Design review of the part built by this model. Coordinates are the model's own, in mm. A direction names the side the tool comes from. Give positions to 0.01 mm unless a question says otherwise; leave off trailing zeros. Loops run counter-clockwise (first coordinate to the right, second up) from the corner with the lowest first, then second, coordinate; pieces in that order, holes last. Notation, with made-up numbers: (45.5, 53) -> (76.5, 53) arc R19 cw to (76.5, 73) -> close; hole circle Ø3 at (47, -9). An arc over 180 degrees is marked (long way). Answer in a Markdown table with one row per item. Add a question column.
(1) Draft analysis for pull direction Y (two halves, no side actions). For faces 1 (the flat face through (-0.1, -15, 2.4)), 2 (the cylindrical face through (3, -42, 0)), state which applies: +Y half, -Y half, draft (parallel to the pull), parting line (faces both ways), or undercut.
(2) Consider section A-A on y = -20.5. Write out the cut boundary in (x, z), then the cut area to 3 significant figures.
(3) Consider section B-B on y = -41. Write out the cut boundary in (x, z), then the cut area to 3 significant figures.
(4) For line 1 (Z direction, x = 0, y = -13.5); line 2 (Z direction, x = 0, y = -32.5); line 3 (X direction, y = -1.5, z = -5.5), list the stretches that pass through material, from the lowest coordinate up.
(5) For pin 1 (8 mm diameter, centred on x = -5.5, y = -15.5, fed in from -Z); pin 2 (1.5 mm diameter, centred on y = -34.5, z = 3, fed in from -X); pin 3 (1.5 mm diameter, centred on x = 6.5, y = -9.5, fed in from -Z), all flat-tipped, find the tip position at first contact; note any pin that passes through.
(6) For faces 3 (the cylindrical face through (-2.17, -32.49, -9.76)), 4 (the cylindrical face through (0.434, -35.493, 1.952)), list the 3-axis set-ups (+Z, -Z, +X, -X, +Y, -Y) from which the entire face can be reached by the end or side of a thin tool; tool diameter is ignored.
from build123d import *

# Parameters (mm, degrees)
ESQUISSE3_R                = 10
ESQUISSE3_R_2              = 2
BOSS_EXTRU_1_DEPTH         = 1
R_P_TITION_LIN_AIRE1_COUNT = 15
R_P_TITION_LIN_AIRE1_PITCH = 2
CHANFREIN1_SIZE            = 1
CHANFREIN1_SIZE2           = 1.732050808
CHANFREIN3_SIZE            = 0.5


with BuildPart() as part:
    # Esquisse2 → Révolution1 (revolve)
    with BuildSketch(Plane.XY):
        Polygon((-1, 0), (-1, -44), (-3, -44), (-3, -40), (-2, -40), (-2, -10), (-8, -10), (-8, -7.5), (-4.5, -6), (-4.5, -4), (-8, -2.5), (-8, 0), align=None)
    revolve(axis=Axis((0, 9.191211929, 0), (0, -1, 0)))

    # Esquisse3 → Boss.-Extru.1 (add)
    with BuildSketch(Plane.XZ.offset(10)):
        Circle(ESQUISSE3_R)
        Circle(ESQUISSE3_R_2, mode=Mode.SUBTRACT)
    boss_extru_1 = extrude(amount=BOSS_EXTRU_1_DEPTH)

    # Répétition linéaire1: Boss.-Extru.1 ×15
    with Locations(*[(0, -i * R_P_TITION_LIN_AIRE1_PITCH, 0) for i in range(1, R_P_TITION_LIN_AIRE1_COUNT)]):
        add(boss_extru_1)

    # Chanfrein1
    chanfrein1_edges = [part.edges().sort_by_distance(p)[0] for p in [
        (1, 0, 0),
    ]]
    chanfrein1_side = [part.faces().sort_by_distance(p)[0] for p in [
        (7.77372583, 0, 0),
    ]]
    chamfer(chanfrein1_edges, length=CHANFREIN1_SIZE, length2=CHANFREIN1_SIZE2, reference=chanfrein1_side[0])

    # Chanfrein3
    chanfrein3_edges = [part.edges().sort_by_distance(p)[0] for p in [
        (3, -40, 0),
        (3, -44, 0),
    ]]
    chamfer(chanfrein3_edges, length=CHANFREIN3_SIZE)


solid = part.part
Values follow:
| question | item | result |
|---|---|---|
| 1 | face 1 | undercut |
| 1 | face 2 | draft |
| 2 | outline | circle Ø20 at (0, 0); hole circle Ø2 at (0, 0) |
| 2 | area | 311 mm2 |
| 3 | outline | circle Ø6 at (0, 0); hole circle Ø2 at (0, 0) |
| 3 | area | 25.1 mm2 |
| 4 | line 1 | -2 to -1, 1 to 2 |
| 4 | line 2 | -10 to -1, 1 to 10 |
| 4 | line 3 | -5.81 to 5.81 |
| 5 | pin 1 | z = -9.88 |
| 5 | pin 2 | x = -9.74 |
| 5 | pin 3 | z = -8.04 |
| 6 | face 3 | +Y, -Y |
| 6 | face 4 | none |
